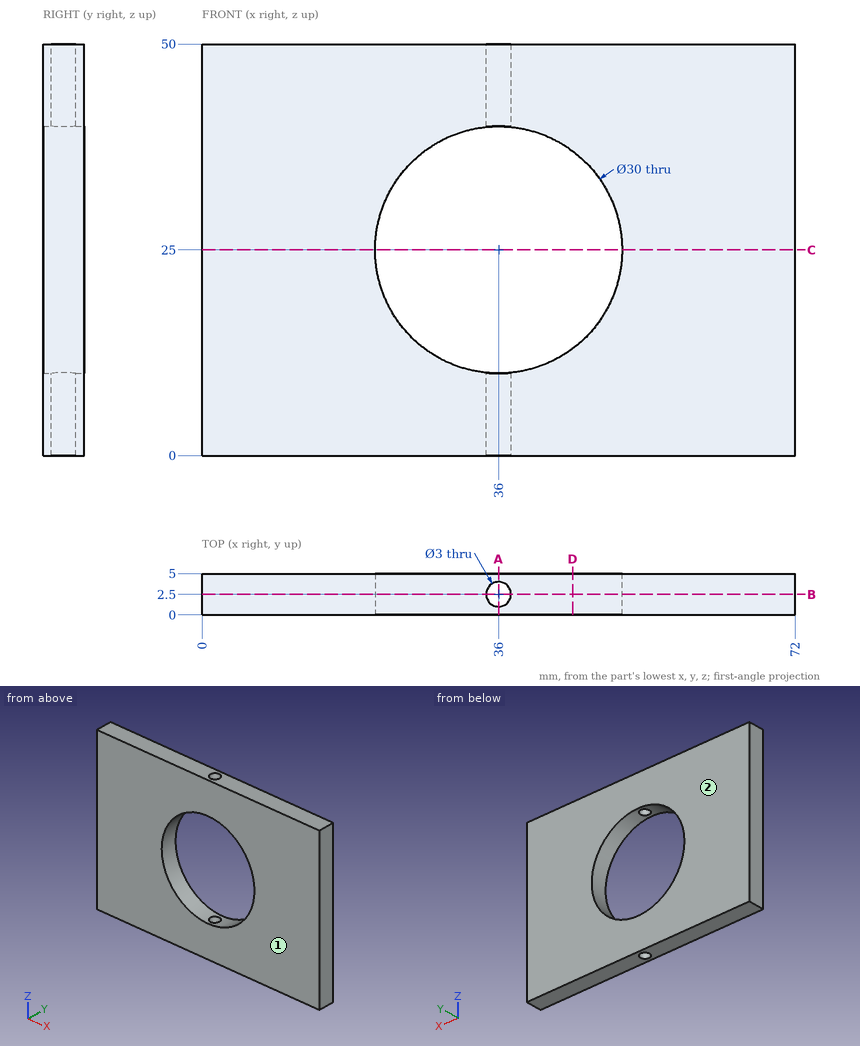
Could you check a few things on this drawing? It's one solid part, dimensions in mm from its lowest x, y, z. Coordinates: 2 decimals unless noted, no trailing zeros. Order: outer loops, then holes, each group sorted by start corner. A loop starts at its lowest first (then second) coordinate and runs counter-clockwise, first axis right, second up. Notation, with made-up numbers: (-2.5, -36.75) - (10.5, -36.75) arc R20 cw to (10.5, -6.75) - close; hole circle Ø7 at (-39.5, -13). An arc over 180 degrees is marked (long way). Answer as a JSON object with one key per item and string values. Group by question number.
Q1. We'd pull the mould along Y, two halves only. Please class the marked faces 1 and 2: +Y half, -Y half, draft (parallel to the pull), parting line (faces both ways), or undercut.
Q2. Imagine slicing it at A-A (x = 36). Please give me the cut outline in (y, z).
Q3. I need wall thicknesses on line 1 (Y direction, x = 36, z = 2); line 2 (X direction, y = 2.45, z = 9); line 3 (Z direction, x = 23.5, y = 2.45). Which ranges of each line are inside material? Lowest first, please. Write a range as from..to.
Q4. Imagine slicing it at C-C (z = 25). Please give me the cut outline in (x, y), and give its area (3 significant figures).
Q5. Imagine slicing it at D-D (x = 45). Please give me the cut outline in (y, z).
Q6. Imagine slicing it at B-B (y = 2.5). Please give me the cut outline in (x, z), and give its area (3 significant figures).
Determined:
{
 "1": {"face 1": "-Y half", "face 2": "+Y half"},
 "2": {"outline": "(0, 0) - (1, 0) - (1, 10) - (0, 10) - close; (0, 40) - (1, 40) - (1, 50) - (0, 50) - close; (4, 0) - (5, 0) - (5, 10) - (4, 10) - close; (4, 40) - (5, 40) - (5, 50) - (4, 50) - close"},
 "3": {"line 1": "y = 0..1, 4..5", "line 2": "x = 0..34.5, 37.5..72", "line 3": "z = 0..16.71, 33.29..50"},
 "4": {"outline": "(0, 0) - (21, 0) - (21, 5) - (0, 5) - close; (51, 0) - (72, 0) - (72, 5) - (51, 5) - close", "area": "210 mm2"},
 "5": {"outline": "(0, 0) - (5, 0) - (5, 13) - (0, 13) - close; (0, 37) - (5, 37) - (5, 50) - (0, 50) - close"},
 "6": {"outline": "(0, 0) - (34.5, 0) - (34.5, 10.08) arc R15 cw to (34.5, 39.92) - (34.5, 50) - (0, 50) - close; (37.5, 0) - (72, 0) - (72, 50) - (37.5, 50) - (37.5, 39.92) arc R15 cw to (37.5, 10.08) - close", "area": "2,830 mm2"}
}
